Autodesk Fusion 360 part; units mm, degrees
sketch "Sketch1" plane through (0, 0, 0) normal (0, 0, 1) x (1, 0, 0)
  line L0 (20, 12.5) -> (-20, 12.5)
  line L1 (-20, 12.5) -> (-20, -12.5)
  line L2 (-20, -12.5) -> (20, -12.5)
  line L3 (20, -12.5) -> (20, 12.5)
  line L4 (20, 12.5) -> (-20, -12.5) construction
  line L5 (-20, 12.5) -> (20, -12.5) construction
  line L6 (-15.05, -12.5) -> (-15.05, -2.5)
  line L7 (-15.05, -2.5) -> (-6.05, -2.5)
  line L8 (0, 12.5) -> (0, -12.5) construction
  line L9 (-6.05, -2.5) -> (-6.05, 6)
  line L10 (-6.05, 6) -> (0, 6)
  line L11 (15.05, -12.5) -> (15.05, -2.5)
  line L12 (15.05, -2.5) -> (6.05, -2.5)
  line L13 (6.05, -2.5) -> (6.05, 6)
  line L14 (6.05, 6) -> (0, 6)
  dimension "d1" = 40
  dimension "d2" = 25
  dimension "d3" = 15.05
  dimension "d4" = 10
  dimension "d5" = 6.05
  dimension "d6" = 8.5
extrude "Extrude1" add sketch "Sketch1" along normal blind 8 contours L0 L1 L2 L3 L6 L7 L9 L10 L11 L12 L13 L14
fillet "Fillet1" radius 5 2 edges at (-20, 12.5, 4) (20, 12.5, 4)
fillet "Fillet2" radius 1 4 edges at (-6.05, -2.5, 4) (6.05, -2.5, 4) (-15.05, -12.5, 4) (15.05, -12.5, 4)
chamfer "Chamfer2" distance 0.4 angle 45 40 edges at (6.05, 2.25, 0) (6.3429, -2.2071, 0) (11.05, -2.5, 0) (0, 6, 0) (-11.05, -2.5, 0) (-6.3429, -2.2071, 0) (-6.05, 2.25, 0) (-18.025, -12.5, 0) (-15.3429, -12.2071, 0) (-15.05, -7, 0) (15.05, -7, 0) (15.3429, -12.2071, 0) (18.025, -12.5, 0) (20, -12.5, 4) (18.025, -12.5, 8) (15.3429, -12.2071, 8) (15.05, -7, 8) (-20, -12.5, 4) (-15.05, -7, 8) (-15.3429, -12.2071, 8) (-18.025, -12.5, 8) (-6.05, 2.25, 8) (-6.3429, -2.2071, 8) (-11.05, -2.5, 8) (0, 6, 8) (11.05, -2.5, 8) (6.3429, -2.2071, 8) (6.05, 2.25, 8) (20, -2.5, 8) (18.5355, 11.0355, 8) (0, 12.5, 8) (-18.5355, 11.0355, 8) (-20, -2.5, 8) (20, -2.5, 0) (18.5355, 11.0355, 0) (0, 12.5, 0) (-18.5355, 11.0355, 0) (-20, -2.5, 0) (-15.05, -2.5, 4) (15.05, -2.5, 4)
Check sheet for the modelled part. Datum: model origin and axes. Units: mm. A direction names the side the tool comes from. Round coordinates to 2 decimals unless told otherwise and drop trailing zeros. Order: outer loops, then holes, each group sorted by start corner. A loop starts at its lowest first (then second) coordinate and runs counter-clockwise, first axis right, second up. Notation, with made-up numbers: M 72,32 L 102,32 A36 cw 102,70 Z; hole C 3,69 d1. An arc over 180 degrees is marked long. One line per item, written item: value. Start each with the question number.
1. Section check A-A on y = 1. Enter the section's corners in (x, z).
2. Scan lines: line 1 along X through (y, z) = (0.5, 1); line 2 along X through (y, z) = (-8.75, 6); line 3 along Y through (x, z) = (11, 7.5). Record each from-to range of solid material in increasing order.
3. Section check C-C on z = 2.75. Enter the section's corners in (x, y), and give its area (3 significant figures).
4. Section check D-D on y = -9.5. Enter the section's corners in (x, z), and give its area (3 significant figures).
5. Gauge pin test, flat end, axial feed: P1, Ø2, axis at x = -12.5, z = 5, coming from the -Y side. Record the tip position at first contact, or that the pin passes through.
6. Section check B-B on x = 1. Enter the section's corners in (y, z), and give its area (3 significant figures).
7. Access from +Z, -Z, +X, -X, +Y, -Y to the whole of each face (thin tool, end or side, straight path). Record for faces 1 (the conical face through (-15.52, -12.042, 0.158)), 2 (the flat face through (-11, -2.5, 4)), 3 (the conical face through (6.52, -2.042, 7.842)), 4 (the flat face through (0, 8, 8)), 5 (the flat face through (-18, -12.5, 4)).
Results found:
1. outline: M -20,0.4 L -19.6,0 L -6.45,0 L -6.05,0.4 L -6.05,7.6 L -6.45,8 L -19.6,8 L -20,7.6 Z; M 6.05,0.4 L 6.45,0 L 19.6,0 L 20,0.4 L 20,7.6 L 19.6,8 L 6.45,8 L 6.05,7.6 Z
2. line 1: -20 to -6.05, 6.05 to 20
2. line 2: -20 to -15.05, 15.05 to 20
2. line 3: -2.5 to 12.5
3. outline: M -20,-12.1 L -19.6,-12.5 L -16.05,-12.5 A1 ccw -15.05,-11.5 L -15.05,-2.9 L -14.65,-2.5 L -7.05,-2.5 A1 ccw -6.05,-1.5 L -6.05,6 L 6.05,6 L 6.05,-1.5 A1 ccw 7.05,-2.5 L 14.65,-2.5 L 15.05,-2.9 L 15.05,-11.5 A1 ccw 16.05,-12.5 L 19.6,-12.5 L 20,-12.1 L 20,7.5 A5 ccw 15,12.5 L -15,12.5 A5 ccw -20,7.5 Z
3. area: 585 mm^2
4. outline: M -20,0.4 L -19.6,0 L -15.45,0 L -15.05,0.4 L -15.05,7.6 L -15.45,8 L -19.6,8 L -20,7.6 Z; M 15.05,0.4 L 15.45,0 L 19.6,0 L 20,0.4 L 20,7.6 L 19.6,8 L 15.45,8 L 15.05,7.6 Z
4. area: 78.6 mm^2
5. P1: y = -2.5
6. outline: M 6,0.4 L 6.4,0 L 12.1,0 L 12.5,0.4 L 12.5,7.6 L 12.1,8 L 6.4,8 L 6,7.6 Z
6. area: 51.7 mm^2
7. face 1: -Z, -Y
7. face 2: +Z, -Z, -Y
7. face 3: +Z, -Y
7. face 4: +Z, +X, -X, +Y, -Y
7. face 5: +Z, -Z, +X, -X, -Y
